```python
from build123d import *

# Parameters (mm, degrees)
SKETCH1_R             = 25.1714
SKETCH1_R_2           = 18.8214
BOSS_EXTRUDE1_DEPTH   = 9.906
SKETCH2_R             = 28.575
BOSS_EXTRUDE2_DEPTH   = 5.08
CUT_EXTRUDE1_START    = 3.6322
SKETCH3_R             = 25.1714
SKETCH3_R_2           = 23.3172
CUT_EXTRUDE1_DEPTH    = 3.6322
SKETCH5_W             = 1.778
SKETCH5_H             = 12.5603
SKETCH6_R             = 16.51
CUT_EXTRUDE2_DEPTH    = 44.100364801
SKETCH10_W            = 1.8796
SKETCH10_H            = 3.5052
BOSS_EXTRUDE3_START   = -5.715
SKETCH7_R             = 38.1
SKETCH7_R_2           = 28.575
BOSS_EXTRUDE3_DEPTH   = 5.715
F_6_CLEARANCE_HOLE1_D = 3.6576
CIRPATTERN1_COUNT     = 3
CHAMFER1_SIZE         = 0.508
CHAMFER3_SIZE         = 1.016


with BuildPart() as part:
    # Sketch1 → Boss-Extrude1 (new body)
    with BuildSketch(Plane.XY):
        Circle(SKETCH1_R)
        Circle(SKETCH1_R_2, mode=Mode.SUBTRACT)
    extrude(amount=-BOSS_EXTRUDE1_DEPTH)

    # Sketch2 → Boss-Extrude2 (add)
    with BuildSketch(Plane(origin=(0, 0, -9.906), x_dir=(-1, 0, 0), z_dir=(0, 0, -1))):
        Circle(SKETCH2_R)
    extrude(amount=BOSS_EXTRUDE2_DEPTH)

    # Sketch3 → Cut-Extrude1 (cut)
    with BuildSketch(Plane.XY.offset(-6.731).offset(CUT_EXTRUDE1_START)):
        Circle(SKETCH3_R)
        Circle(SKETCH3_R_2, mode=Mode.SUBTRACT)
    extrude(amount=-CUT_EXTRUDE1_DEPTH, mode=Mode.SUBTRACT)

    # Sketch4 → Revolve1 (revolve)
    with BuildSketch(Plane(origin=(0, 0, 0), x_dir=(0, 0, -1), z_dir=(1, 0, 0)), mode=Mode.PRIVATE) as revolve1_sk:
        Polygon((9.906, 16.51), (9.906, 28.575), (26.416, 28.575), (26.416, 24.0665), (15.621, 24.0665), (15.621, 16.51), align=None)
    revolve(revolve1_sk.sketch.rotate(Axis((0, 0, -23.632862863), (0, 0, 1)), 90), axis=Axis((0, 0, -23.632862863), (0, 0, 1)))

    # Sketch5 → Cut-Revolve1 (revolve, cut)
    with BuildSketch(Plane(origin=(0, 0, 0), x_dir=(0, 0, -1), z_dir=(1, 0, 0)), mode=Mode.PRIVATE) as cut_revolve1_sk:
        with Locations((22.7838, 18.98015)):
            Rectangle(SKETCH5_W, SKETCH5_H)
    revolve(cut_revolve1_sk.sketch.rotate(Axis((0, 0, -23.632862863), (0, 0, 1)), 90), axis=Axis((0, 0, -23.632862863), (0, 0, 1)), mode=Mode.SUBTRACT)

    # Sketch6 → Cut-Extrude2 (cut, through all)
    with BuildSketch(Plane(origin=(0, 0, -14.986), x_dir=(-1, 0, 0), z_dir=(0, 0, -1))):
        Circle(SKETCH6_R)
    extrude(amount=-CUT_EXTRUDE2_DEPTH, mode=Mode.SUBTRACT)

    # Sketch10 → Cut-Revolve2 (revolve, cut)
    with BuildSketch(Plane(origin=(0, 0, 0), x_dir=(0, 0, -1), z_dir=(1, 0, 0)), mode=Mode.PRIVATE) as cut_revolve2_sk:
        with Locations((14.6812, 21.4249)):
            Rectangle(SKETCH10_W, SKETCH10_H)
    revolve(cut_revolve2_sk.sketch.rotate(Axis((0, 0, 0), (0, 0, -1)), 90), axis=Axis((0, 0, 0), (0, 0, -1)), mode=Mode.SUBTRACT)

    # Sketch7 → Boss-Extrude3 (add)
    with BuildSketch(Plane(origin=(0, 0, -15.621), x_dir=(-1, 0, 0), z_dir=(0, 0, -1)).offset(BOSS_EXTRUDE3_START)):
        Circle(SKETCH7_R)
        Circle(SKETCH7_R_2, mode=Mode.SUBTRACT)
    extrude(amount=BOSS_EXTRUDE3_DEPTH)

    # #6 Clearance Hole1 (through all)
    with Locations(Plane(origin=(12.683965444, 15.420187154, -15.621), x_dir=(-1, 0, 0), z_dir=(0, 0, -1))):
        with Locations((12.683965444, 17.917312846)):
            f_6_clearance_hole1 = Hole(F_6_CLEARANCE_HOLE1_D / 2)

    # CirPattern1: #6 Clearance Hole1 ×3 about axis
    cirpattern1_axis = Axis((0, 0, 0), (0, 0, 1))
    for i in range(1, CIRPATTERN1_COUNT):
        add(f_6_clearance_hole1.rotate(cirpattern1_axis, i * 360 / CIRPATTERN1_COUNT), mode=Mode.SUBTRACT)

    # Chamfer1
    chamfer1_edges = [part.edges().sort_by_distance(p)[0] for p in [
        (-25.1714, 0, 0),
        (28.575, 0, -26.416),
        (38.1, 0, -15.621),
        (-18.8214, 0, 0),
    ]]
    chamfer(chamfer1_edges, length=CHAMFER1_SIZE)

    # Chamfer3
    chamfer3_edges = [part.edges().sort_by_distance(p)[0] for p in [
        (24.0665, 0, -26.416),
    ]]
    chamfer(chamfer3_edges, length=CHAMFER3_SIZE)


solid = part.part
```
Build history of the part. All positions in model axes, mm. A direction names the side the tool comes from. Give positions to 0.01 mm unless a question says otherwise; leave off trailing zeros. Write item = value, one per line. Start each with the question number.
(1) Pin check, flat tips, straight feed: pin 1 Ø15 at (x, y) = (9.5, 8.5) entering from -Z; pin 2 Ø2 at (y, z) = (-15.5, -22.5) entering from -X; pin 3 Ø4 at (y, z) = (22.5, -9) entering from +X; pin 4 Ø6 at (x, y) = (-29.5, 8.5) entering from -Z. Stop position of each tip, or through.
(2) Two-plate mould, pull along Y, no slides. Class faces 1 (the cylindrical face through (28.547, 1.256, -20.692)), 2 (the cylindrical face through (-30.322, -17.782, -12.723)), 3 (the flat face through (21, 14, -26.416)): released by +Y, released by -Y, zero draft, split by the parting line, or undercut.
(3) Probe L1, parallel to Y at x = 0, z = -14.4; L2, parallel to Y at x = 0, z = -19 (1 decimal); L3, parallel to Z at x = 17, y = 13.5. List the from-to ranges inside material, lowest first. Write a range as [from, to].
(4) Which spindle directions (+Z, -Z, +X, -X, +Y, -Y) get a long thin tool onto all of the face, cutting with end or side? Do faces 4 (the cylindrical face through (30.235, -23.183, -12.473)), 5 (the cylindrical face through (23.252, -9.641, -1.785)), 6 (the flat face through (25.24, -13.75, -15.621)), 7 (the flat face through (20.5, 13, -23.673)). Say none if no direction does.
(5) Slice it at B-B on x = 0. State how many separate pieces and enclosed holes the cut face has, plus the area to 3 significant figures.
Responses:
q1.pin_1 = -15.62
q1.pin_2 = -24.62
q1.pin_3 = 31.98
q1.pin_4 = -26.42
q2.face_1 = split by the parting line
q2.face_2 = undercut
q2.face_3 = zero draft
q3.L1 = [-38.1, -23.18], [-19.67, -16.51], [16.51, 19.67], [23.18, 31.51], [35.17, 38.1]
q3.L2 = [-28.6, -24.1], [24.1, 28.6]
q3.L3 = [-13.74, 0]
q4.face_4 = +Z, -Z
q4.face_5 = +Z
q4.face_6 = -Z
q4.face_7 = none
q5.separate_pieces = 3
q5.enclosed_holes = 0
q5.area = 416 mm2
